Could you check a few things on this drawing? It's one solid part, dimensions in mm from its lowest x, y, z. A direction names the side the tool comes from. Round coordinates to 2 decimals unless told otherwise and drop trailing zeros. Loops run counter-clockwise (first coordinate to the right, second up) from the corner with the lowest first, then second, coordinate; pieces in that order, holes last. Notation, with made-up numbers: (66.25, 58.5) -> (99.25, 58.5) arc R27 ccw to (99.25, 87.5) -> close; hole circle Ø11 at (8, 8.5). An arc over 180 degrees is marked (long way). Put each result on its own line as item: value. Start each with the question number.
1. Imagine slicing it at B-B, the plane y = 76.2. Please give me the cut outline in (x, z) (3 decimals), and give its area (3 significant figures).
2. I need wall thicknesses on line 1 (Z direction, x = 1, y = 152); line 2 (Z direction, x = 1.5, y = 177.8) (3 decimals); line 3 (X direction, y = 38.1, z = 1.6). Which ranges of each line are inside material? Lowest first, please. Write a range as [from, to].
3. I'm going to push flat-ended pins straight in: P1, Ø3.5, axis at y = 113.5, z = 2, coming from the +X side (3 decimals); P2, Ø10, axis at y = 152.5, z = 5.5, coming from the +X side (3 decimals); P3, Ø14.5, axis at x = 36.5, y = 69, coming from the +Z side (3 decimals). Where does each tip first touch, or does it pass through?
4. Which directions (+Z, -Z, +X, -X, +Y, -Y) give clear straight access to the entire face, cutting with the end or side of a thin tool? Please do the marked faces 1 and 2.
5. Imagine slicing it at D-D, the plane x = 44.5. Please give me the cut outline in (y, z) (3 decimals).
6. Imagine slicing it at C-C, the plane y = 177.8. Please give me the cut outline in (x, z) (3 decimals), and give its area (3 significant figures).
7. Imagine slicing it at A-A, the plane y = 12.7. Please give me the cut outline in (x, z) (3 decimals), and give its area (3 significant figures).
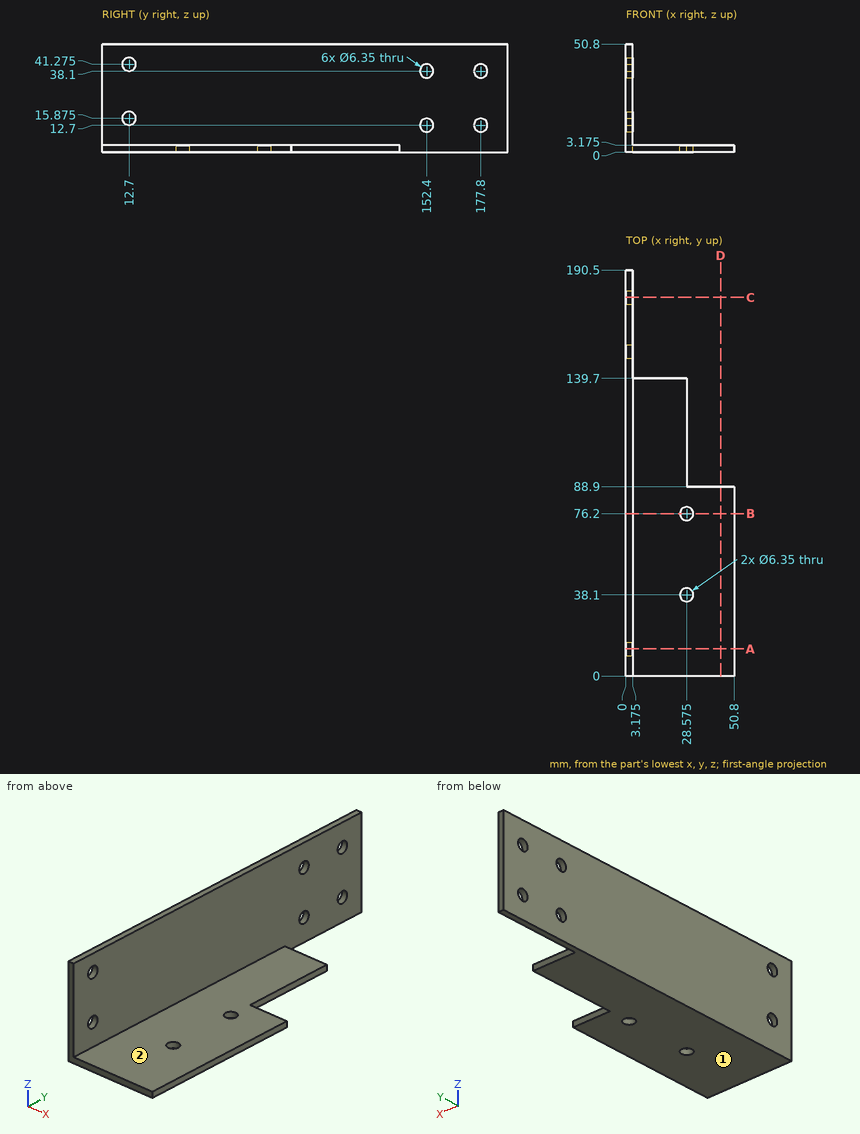
Entries:
1. outline: (0, 0) -> (25.4, 0) -> (25.4, 3.175) -> (3.175, 3.175) -> (3.175, 50.8) -> (0, 50.8) -> close; (31.75, 0) -> (50.8, 0) -> (50.8, 3.175) -> (31.75, 3.175) -> close
1. area: 292 mm^2
2. line 1: [0, 9.55], [15.85, 34.95], [41.25, 50.8]
2. line 2: [0, 9.525], [15.875, 34.925], [41.275, 50.8]
2. line 3: [0, 25.4], [31.75, 50.8]
3. P1: x = 28.575
3. P2: x = 3.175
3. P3: z = 3.175
4. face 1: -Z, +X, -X, +Y, -Y
4. face 2: +Z, +X, +Y, -Y
5. outline: (0, 0) -> (88.9, 0) -> (88.9, 3.175) -> (0, 3.175) -> close
6. outline: (0, 0) -> (3.175, 0) -> (3.175, 9.525) -> (0, 9.525) -> close; (0, 15.875) -> (3.175, 15.875) -> (3.175, 34.925) -> (0, 34.925) -> close; (0, 41.275) -> (3.175, 41.275) -> (3.175, 50.8) -> (0, 50.8) -> close
6. area: 121 mm^2
7. outline: (0, 0) -> (50.8, 0) -> (50.8, 3.175) -> (3.175, 3.175) -> (3.175, 12.7) -> (0, 12.7) -> close; (0, 19.05) -> (3.175, 19.05) -> (3.175, 38.1) -> (0, 38.1) -> close; (0, 44.45) -> (3.175, 44.45) -> (3.175, 50.8) -> (0, 50.8) -> close
7. area: 272 mm^2
